Check sheet for the modelled part. Datum: model origin and axes. Units: mm. A direction names the side the tool comes from. Give positions to 0.01 mm unless a question says otherwise; leave off trailing zeros. Loops run counter-clockwise (first coordinate to the right, second up) from the corner with the lowest first, then second, coordinate; pieces in that order, holes last. Notation, with made-up numbers: (53.5, 44.5) - (112.5, 44.5) arc R18 ccw to (112.5, 54.5) - close; hole circle Ø11 at (38.5, 77.5). An arc over 180 degrees is marked (long way). Answer in a Markdown table with one row per item. Add a question column.
(1) Thickness scan on L1, parallel to X at y = 4.8, z = -174; L2, parallel to Z at x = -150, y = 4.55; L3, parallel to Z at x = -135.5, y = 3.25. Record the ranges inside material, lowest first.
(2) Draft check along X on faces 4 (the face through (-120.13, 2.46, -175.57)), 5 (the face through (-103, 2, -122.182)), 6 (the face through (-79.708, 2.535, -201.335)). Enter one of: released by +X, released by -X, zero draft, split by the parting line, or undercut.
(3) Go/stop test with flat-tipped pins: P1, Ø1.2, axis at x = -71.4, z = -128.19, coming from the +Y side; P2, Ø1.5, axis at x = -56.5, y = 3, coming from the -Z side; P3, Ø1.5, axis at y = 4, z = -160, coming from the +X side; P4, Ø2.5, axis at y = 3.5, z = -181.5, coming from the -X side. Record where each tip stops, or that it passes through.
(4) Sectioned sample at C-C on y = 4.15. State how many separate pieces and enclosed holes the cut face has, then the cut area to 3 significant figures.
(5) Sectioned sample at B-B on z = -130.5. Enter the section's corners in (x, y), then the cut area to 3 significant figures.
(6) Set-up check for faces 1 (the face through (-144, 3, -133.287)), 2 (the face through (-107.55, 2.46, -147.3)), 3 (the face through (-128.853, 2, -176)): record each of +Z, -Z, +X, -X, +Y, -Y from which the full face is reachable in a straight line by a thin tool's end or side.
(7) Sectioned sample at A-A on z = -158. Enter the section's corners in (x, y), then the cut area to 3 significant figures.
from build123d import *

# Parameters (mm, degrees)
EXTRUDE_4_DEPTH      = 5
EXTRUDE_5_DEPTH      = 5
EXTRUDE_6_DEPTH      = 5
SKETCH_5_R           = 1.7
CUT_EXTRUDE_1_DEPTH  = 5
EXTRUDE_7_DEPTH      = 5
SKETCH_7_R           = 1.7
CUT_EXTRUDE_2_DEPTH  = 5
SKETCH_12_W          = 15
SKETCH_12_H          = 3
EXTRUDE_10_DEPTH     = 5
CUT_EXTRUDE_5_DEPTH  = 5
SKETCH_14_W          = 15
SKETCH_14_H          = 5
EXTRUDE_11_DEPTH     = 5
SKETCH_16_R          = 2.2
CUT_EXTRUDE_7_DEPTH  = 5
CUT_EXTRUDE_8_DEPTH  = 5
SKETCH_19_R          = 2.2
CUT_EXTRUDE_9_DEPTH  = 5
EXTRUDE_12_DEPTH     = 5
FILLET_1_R           = 2
SKETCH_21_W          = 134.232837099
SKETCH_21_H          = 189.007158486
SKETCH_21_W_2        = 166.269417525
SKETCH_21_H_2        = 176.352735834
CUT_EXTRUDE_10_DEPTH = 314.073605795
SKETCH_22_W          = 20
SKETCH_22_H          = 60
SKETCH_22_R          = 2.1
EXTRUDE_13_DEPTH     = 5
FILLET_2_R           = 10
FILLET_3_R           = 3


with BuildPart() as part:
    # Sketch 2 → Extrude 4 (new body)
    with BuildSketch(Plane(origin=(0, 0, 0), x_dir=(1, 0, 0), z_dir=(0, 1, 0))):
        Polygon((-163.852515924, 124.182366776), (-43.852515924, 124.182366776), (16.242365952, 59.136369948), (32.045701527, 59.136369948), (51.147484076, 9.582366776), (51.147484076, -23.417633224), (71.147484076, -23.417633224), (71.147484076, 11.582366776), (41.16464964, 70.136369948), (23.597046938, 70.136369948), (-38.39605211, 137.236974827), (-169.308979739, 137.236974827), (-231.302078787, 70.136369948), (-248.869681489, 70.136369948), (-278.852515924, 11.582366776), (-278.852515924, -23.417633224), (-258.852515924, -23.417633224), (-258.852515924, 9.582366776), (-239.750733376, 59.136369948), (-223.947397801, 59.136369948), align=None)
    extrude(amount=EXTRUDE_4_DEPTH)

    # Sketch 3 → Extrude 5 (add)
    with BuildSketch(Plane(origin=(0, 5, 0), x_dir=(1, 0, 0), z_dir=(0, 1, 0))):
        Polygon((-258.852515924, -23.417633224), (-252.852515924, -23.417633224), (-252.852515924, 16.806798308), (-236.535564294, 59.136369948), (-239.750733376, 59.136369948), (-258.852515924, 9.582366776), align=None)
        Polygon((51.147484076, -23.417633224), (45.147484076, -23.417633224), (45.147484076, 16.806798308), (28.830532445, 59.136369948), (32.045701527, 59.136369948), (51.147484076, 9.582366776), align=None)
    extrude(amount=-EXTRUDE_5_DEPTH)

    # Sketch 4 → Extrude 6 (add)
    with BuildSketch(Plane(origin=(0, 5, 0), x_dir=(1, 0, 0), z_dir=(0, 1, 0))):
        Polygon((-252.852515924, 16.806798308), (-244.852515924, -15.417633224), (-244.852515924, -23.417633224), (-252.852515924, -23.417633224), align=None)
    extrude(amount=-EXTRUDE_6_DEPTH)

    # Sketch 5 → Cut-Extrude 1 (cut)
    with BuildSketch(Plane.XZ):
        with Locations(Location((-273.852515924, 19.417633224, 0), (0, 0, 270))):
            Circle(SKETCH_5_R)
        with Locations(Location((-257.852515924, 19.417633224, 0), (0, 0, 270))):
            Circle(SKETCH_5_R)
    extrude(amount=-CUT_EXTRUDE_1_DEPTH, mode=Mode.SUBTRACT)

    # Sketch 6 → Extrude 7 (add)
    with BuildSketch(Plane(origin=(0, 5, 0), x_dir=(1, 0, 0), z_dir=(0, 1, 0))):
        Polygon((45.147484076, -23.417633224), (37.147484076, -23.417633224), (37.147484076, -15.417633224), (45.147484076, 16.806798308), align=None)
    extrude(amount=-EXTRUDE_7_DEPTH)

    # Sketch 7 → Cut-Extrude 2 (cut)
    with BuildSketch(Plane.XZ):
        with Locations(Location((66.147484076, 19.417633224, 0), (0, 0, 270))):
            Circle(SKETCH_7_R)
        with Locations(Location((50.147484076, 19.417633224, 0), (0, 0, 270))):
            Circle(SKETCH_7_R)
    extrude(amount=-CUT_EXTRUDE_2_DEPTH, mode=Mode.SUBTRACT)

    # Sketch 13 → Cut-Extrude 5 (cut)
    with BuildSketch(Plane(origin=(0, 5, 0), x_dir=(1, 0, 0), z_dir=(0, 1, 0))):
        with BuildLine():
            Line((-253.852515924, -23.417633224), (-251.852515924, -23.417633224))
            ThreePointArc((-251.852515924, -23.417633224), (-252.852515924, -22.417633224), (-253.852515924, -23.417633224))
        make_face()
        with BuildLine():
            Line((-268.852515924, -23.417633224), (-270.852515924, -23.417633224))
            ThreePointArc((-270.852515924, -23.417633224), (-269.852515924, -22.417633224), (-268.852515924, -23.417633224))
        make_face()
    cut_extrude_5 = extrude(amount=-CUT_EXTRUDE_5_DEPTH, mode=Mode.SUBTRACT)



with BuildPart() as body_2:
    # Sketch 12 → Extrude 10 (new body)
    with BuildSketch(Plane(origin=(0, 5, 0), x_dir=(1, 0, 0), z_dir=(0, 1, 0))):
        with Locations((-261.352515924, -24.917633224)):
            Rectangle(SKETCH_12_W, SKETCH_12_H)
    extrude(amount=-EXTRUDE_10_DEPTH)


with BuildPart() as part_1:
    add(part.part)

    add(body_2.part)  # Extrude 11 merges body 2
    # Sketch 14 → Extrude 11 (add)
    with BuildSketch(Plane.XY.offset(26.417633224)):
        with Locations((-261.352515924, 2.5)):
            Rectangle(SKETCH_14_W, SKETCH_14_H)
    extrude_11 = extrude(amount=-EXTRUDE_11_DEPTH)

    # Mirror 4: Cut-Extrude 5, Extrude 11 across plane
    add(cut_extrude_5.mirror(Plane.ZY.offset(103.852515924)), mode=Mode.SUBTRACT)
    add(extrude_11.mirror(Plane.ZY.offset(103.852515924)))

    # Sketch 16 → Cut-Extrude 7 (cut)
    with BuildSketch(Plane(origin=(0, 5, 0), x_dir=(1, 0, 0), z_dir=(0, 1, 0))):
        with Locations(Location((-222.724177384, 69.940679724, 0), (0, 0, 270))):
            Circle(SKETCH_16_R)
        with Locations(Location((-182.008197488, 114.011179848, 0), (0, 0, 270))):
            Circle(SKETCH_16_R)
        with Locations(Location((-209.152184085, 84.630846432, 0), (0, 0, 270))):
            Circle(SKETCH_16_R)
        with Locations(Location((1.447152236, 84.630846432, 0), (0, 0, 90))):
            Circle(SKETCH_16_R)
        with Locations(Location((-25.696834361, 114.011179848, 0), (0, 0, 90))):
            Circle(SKETCH_16_R)
        with Locations(Location((15.019145535, 69.940679724, 0), (0, 0, 90))):
            Circle(SKETCH_16_R)
        with Locations(Location((-262.852515924, 20.136369948, 0), (0, 0, 270))):
            Circle(SKETCH_16_R)
        with Locations(Location((55.147484076, 20.136369948, 0), (0, 0, 90))):
            Circle(SKETCH_16_R)
    extrude(amount=-CUT_EXTRUDE_7_DEPTH, mode=Mode.SUBTRACT)

    # Sketch 18 → Cut-Extrude 8 (cut)
    with BuildSketch(Plane(origin=(0, 5, 0), x_dir=(1, 0, 0), z_dir=(0, 1, 0))):
        with BuildLine():
            Line((-151.402515924, 132.286974827), (-151.402515924, 129.186974827))
            ThreePointArc((-151.402515924, 129.186974827), (-152.109622706, 127.479868046), (-150.402515924, 128.186974827))
            Line((-150.402515924, 128.186974827), (-137.302515924, 128.186974827))
            ThreePointArc((-137.302515924, 128.186974827), (-135.595409143, 127.479868046), (-136.302515924, 129.186974827))
            Line((-136.302515924, 129.186974827), (-136.302515924, 132.286974827))
            ThreePointArc((-136.302515924, 132.286974827), (-135.595409143, 133.994081608), (-137.302515924, 133.286974827))
            Line((-137.302515924, 133.286974827), (-150.402515924, 133.286974827))
            ThreePointArc((-150.402515924, 133.286974827), (-152.109622706, 133.994081608), (-151.402515924, 132.286974827))
        make_face()
        with BuildLine():
            Line((-97.302515924, 133.286974827), (-110.402515924, 133.286974827))
            ThreePointArc((-110.402515924, 133.286974827), (-112.109622706, 133.994081608), (-111.402515924, 132.286974827))
            Line((-111.402515924, 132.286974827), (-111.402515924, 129.186974827))
            ThreePointArc((-111.402515924, 129.186974827), (-112.109622706, 127.479868046), (-110.402515924, 128.186974827))
            Line((-110.402515924, 128.186974827), (-97.302515924, 128.186974827))
            ThreePointArc((-97.302515924, 128.186974827), (-95.595409143, 127.479868046), (-96.302515924, 129.186974827))
            Line((-96.302515924, 129.186974827), (-96.302515924, 132.286974827))
            ThreePointArc((-96.302515924, 132.286974827), (-95.595409143, 133.994081608), (-97.302515924, 133.286974827))
        make_face()
        with BuildLine():
            Line((-57.302515924, 133.286974827), (-70.402515924, 133.286974827))
            ThreePointArc((-70.402515924, 133.286974827), (-72.109622706, 133.994081608), (-71.402515924, 132.286974827))
            Line((-71.402515924, 132.286974827), (-71.402515924, 129.186974827))
            ThreePointArc((-71.402515924, 129.186974827), (-72.109622706, 127.479868046), (-70.402515924, 128.186974827))
            Line((-70.402515924, 128.186974827), (-57.302515924, 128.186974827))
            ThreePointArc((-57.302515924, 128.186974827), (-55.595409143, 127.479868046), (-56.302515924, 129.186974827))
            Line((-56.302515924, 129.186974827), (-56.302515924, 132.286974827))
            ThreePointArc((-56.302515924, 132.286974827), (-55.595409143, 133.994081608), (-57.302515924, 133.286974827))
        make_face()
    extrude(amount=-CUT_EXTRUDE_8_DEPTH, mode=Mode.SUBTRACT)

    # Sketch 19 → Cut-Extrude 9 (cut)
    with BuildSketch(Plane.XZ):
        with Locations(Location((-123.852515924, -130.736974827, 0), (0, 0, 270))):
            Circle(SKETCH_19_R)
        with Locations(Location((-83.852515924, -130.736974827, 0), (0, 0, 90))):
            Circle(SKETCH_19_R)
    extrude(amount=-CUT_EXTRUDE_9_DEPTH, mode=Mode.SUBTRACT)

    # Sketch 20 → Extrude 12 (add)
    with BuildSketch(Plane.XZ):
        Polygon((29.601480556, -57.136369948), (15.367221806, -57.136369948), (-44.727660071, -122.182366776), (-162.977371778, -122.182366776), (-223.072253655, -57.136369948), (-237.306512405, -57.136369948), (-236.535564294, -59.136369948), (-223.947397801, -59.136369948), (-163.852515924, -124.182366776), (-43.852515924, -124.182366776), (16.242365952, -59.136369948), (28.830532445, -59.136369948), align=None)
        Polygon((-248.869681489, -70.136369948), (-246.309409534, -75.136369948), (-233.489939153, -75.136369948), (-171.496840105, -142.236974827), (-36.208191744, -142.236974827), (25.784907304, -75.136369948), (38.604377685, -75.136369948), (41.16464964, -70.136369948), (23.597046938, -70.136369948), (-38.39605211, -137.236974827), (-169.308979739, -137.236974827), (-231.302078787, -70.136369948), align=None)
    extrude(amount=-EXTRUDE_12_DEPTH)

    # Fillet 1
    fillet_1_edges = [part_1.edges().sort_by_distance(p)[0] for p in [
        (-278.852515924, 2.5, 23.417633224),
        (71.147484076, 2.5, 23.417633224),
        (-244.852515924, 2.5, 23.417633224),
        (-244.852515924, 2.5, 15.417633224),
        (37.147484076, 2.5, 23.417633224),
        (37.147484076, 2.5, 15.417633224),
    ]]
    fillet(fillet_1_edges, radius=FILLET_1_R)

    # Sketch 21 → Cut-Extrude 10 (cut, through all)
    with BuildSketch(Plane.XZ):
        with Locations((-230.093790328, -47.733395584)):
            Rectangle(SKETCH_21_W, SKETCH_21_H)
        with Locations((38.407048692, -54.06060691)):
            Rectangle(SKETCH_21_W_2, SKETCH_21_H_2)
    extrude(amount=-CUT_EXTRUDE_10_DEPTH, mode=Mode.SUBTRACT)

    # Sketch 22 → Extrude 13 (add, through all)
    # profile 1 of 2: a face of its own
    with BuildSketch(Plane.XZ):
        with Locations((-118.852515924, -172.236974827)):
            Rectangle(SKETCH_22_W, SKETCH_22_H)
        with Locations(Location((-118.852515924, -197.236974827, 0), (0, 0, 270))):
            Circle(SKETCH_22_R, mode=Mode.SUBTRACT)
        with Locations(Location((-118.852515924, -177.236974827, 0), (0, 0, 270))):
            Circle(SKETCH_22_R, mode=Mode.SUBTRACT)
        with Locations(Location((-118.852515924, -157.236974827, 0), (0, 0, 270))):
            Circle(SKETCH_22_R, mode=Mode.SUBTRACT)
    # profile 2 of 2: a face of its own
    with BuildSketch(Plane.XZ):
        with Locations((-88.852515924, -172.236974827)):
            Rectangle(SKETCH_22_W, SKETCH_22_H)
        with Locations(Location((-88.852515924, -197.236974827, 0), (0, 0, 90))):
            Circle(SKETCH_22_R, mode=Mode.SUBTRACT)
        with Locations(Location((-88.852515924, -177.236974827, 0), (0, 0, 90))):
            Circle(SKETCH_22_R, mode=Mode.SUBTRACT)
        with Locations(Location((-88.852515924, -157.236974827, 0), (0, 0, 90))):
            Circle(SKETCH_22_R, mode=Mode.SUBTRACT)
    extrude(amount=-EXTRUDE_13_DEPTH)

    # Fillet 2
    # the kernel refuses this fillet: 10 mm, written as the material it adds along each edge
    with BuildSketch(Plane(origin=(-128.852515924, 0, -142.236974827), x_dir=(-1, 0, 0), z_dir=(0, 1, 0)), Plane(origin=(-98.852515924, 0, -142.236974827), x_dir=(-1, 0, 0), z_dir=(0, 1, 0))) as fillet_2_piece_1:
        with BuildLine():
            CenterArc((FILLET_2_R, -FILLET_2_R), FILLET_2_R, 90, 90)
            Line((0, -FILLET_2_R), (0, 0))
            Line((0, 0), (FILLET_2_R, 0))
        make_face()
    extrude(amount=5)
    with BuildSketch(Plane(origin=(-108.852515924, 0, -142.236974827), x_dir=(1, 0, 0), z_dir=(0, 1, 0)), Plane(origin=(-78.852515924, 0, -142.236974827), x_dir=(1, 0, 0), z_dir=(0, 1, 0))) as fillet_2_piece_2:
        with BuildLine():
            CenterArc((FILLET_2_R, FILLET_2_R), FILLET_2_R, 180, 90)
            Line((0, FILLET_2_R), (0, 0))
            Line((0, 0), (FILLET_2_R, 0))
        make_face()
    extrude(amount=5)

    # Fillet 3
    fillet_3_edges = [part_1.edges().sort_by_distance(p)[0] for p in [
        (-162.977371778, 2.5, -122.182366776),
        (-44.727660071, 2.5, -122.182366776),
        (-162.977371778, 2.5, -142.236974827),
        (-44.727660071, 2.5, -142.236974827),
        (-128.852515924, 2.5, -202.236974827),
        (-108.852515924, 2.5, -202.236974827),
        (-78.852515924, 2.5, -202.236974827),
        (-98.852515924, 2.5, -202.236974827),
    ]]
    fillet(fillet_3_edges, radius=FILLET_3_R)


solid = part_1.part
Reply:
| question | item | result |
|---|---|---|
| 1 | L1 | -128.85 to -108.85, -98.85 to -78.85 |
| 1 | L2 | -142.24 to -133.29, -128.19 to -122.18 |
| 1 | L3 | -142.82 to -133.88, -132.69 to -128.78, -127.59 to -122.18 |
| 2 | face 4 | undercut |
| 2 | face 5 | zero draft |
| 2 | face 6 | released by +X |
| 3 | P1 | through |
| 3 | P2 | z = -142.24 |
| 3 | P3 | x = -78.85 |
| 3 | P4 | x = -128.85 |
| 4 | separate pieces | 1 |
| 4 | enclosed holes | 11 |
| 4 | area | 4,460 mm^2 |
| 5 | outline | (-162.98, 0) - (-151.4, 0) - (-151.4, 5) - (-162.98, 5) - close; (-136.3, 0) - (-126.04, 0) - (-126.04, 5) - (-136.3, 5) - close; (-121.67, 0) - (-111.4, 0) - (-111.4, 5) - (-121.67, 5) - close; (-96.3, 0) - (-86.04, 0) - (-86.04, 5) - (-96.3, 5) - close; (-81.67, 0) - (-71.4, 0) - (-71.4, 5) - (-81.67, 5) - close; (-56.3, 0) - (-44.73, 0) - (-44.73, 5) - (-56.3, 5) - close |
| 5 | area | 321 mm^2 |
| 6 | face 1 | +Y, -Y |
| 6 | face 2 | -Z, +Y, -Y |
| 6 | face 3 | -Z, -X, +Y, -Y |
| 7 | outline | (-128.85, 0) - (-120.81, 0) - (-120.81, 5) - (-128.85, 5) - close; (-116.9, 0) - (-108.85, 0) - (-108.85, 5) - (-116.9, 5) - close; (-98.85, 0) - (-90.81, 0) - (-90.81, 5) - (-98.85, 5) - close; (-86.9, 0) - (-78.85, 0) - (-78.85, 5) - (-86.9, 5) - close |
| 7 | area | 161 mm^2 |
